Autodesk Inventor part; units mm, degrees
ref_plane "YZ Plane" through (0, 0, 0) normal (1, 0, 0) x (0, 1, 0)
ref_plane "XZ Plane" through (0, 0, 0) normal (0, 1, 0) x (-1, 0, 0)
ref_plane "XY Plane" through (0, 0, 0) normal (0, 0, 1) x (1, 0, 0)
sketch "Sketch1" plane through (0, 0, 0) normal (0, 0, 1) x (1, 0, 0)
  line L0 (-23.5606, 6.7424) -> (-13.5606, 6.7424)
  line L1 (-13.5606, 6.7424) -> (-13.5606, -1.2576)
  line L2 (-13.5606, -1.2576) -> (-23.5606, -1.2576)
  line L3 (-23.5606, -1.2576) -> (-23.5606, 6.7424)
  point P0 (0, 0)
  dimension "d0" = 10
  dimension "d1" = 8
extrude "Extrusion1" add sketch "Sketch1" along normal blind 23
sketch "Sketch2" plane through (0, 0, 23) normal (0, 0, 1) x (1, 0, 0)
  line L0 (-23.5606, 6.7424) -> (-23.5606, -1.2576)
  point P0 (0, 0)
  point P1 (-18.5606, 2.7424)
  dimension "d4" = 5
hole "Hole1" at (-18.5606, 2.7424, 23) direction (0, 0, -1) diameter 3 depth 8 tip angle 118
sketch "Sketch3" plane through (-13.5606, -1.2576, 0) normal (1, 0, 0) x (0, 0, -1)
  line L0 (0, 8) -> (-3, 8)
  line L1 (-3, 8) -> (-3, 13)
  line L2 (-3, 13) -> (0, 13)
  line L3 (0, 13) -> (0, 8)
  line L4 (0, 0) -> (-23, 0)
  point P0 (0, 1.2576)
  dimension "d12" = 13
  dimension "d13" = 3
extrude "Extrusion2" add sketch "Sketch3" against normal blind 10
chamfer "Chamfer1" distance 3 angle 45 1 edges at (-18.5606, 6.7424, 3)
properties part number "ArOZ Portable Mount"
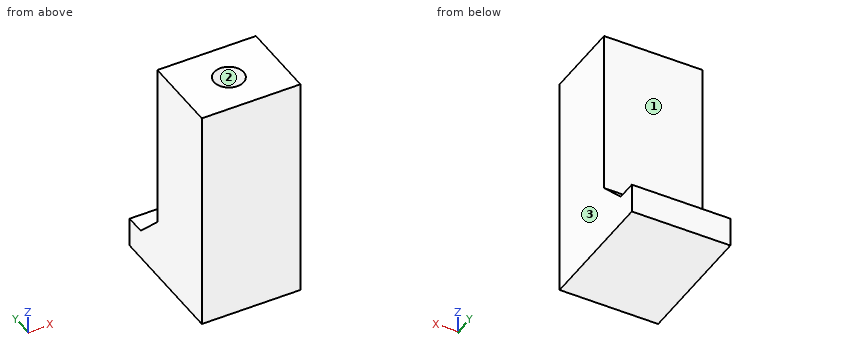
Could you check a few things on this model? Use its own coordinates, in mm. Face numbers are marked on the shaded views. Give positions to 0.01 mm unless a question says otherwise; leave off trailing zeros. Write each loop counter-clockwise with the first axis right and the second up, starting at its lowest first coordinate (ties: lowest second). Pieces come first, ordered by that corner, then holes. Notation, with made-up numbers: (-38, 45) - (-22, 45) arc R27 cw to (-22, 72) - close; hole circle Ø2 at (-40, -28.5). An arc over 180 degrees is marked (long way). Use CSV: the item, a comma, the result in double quotes. Start each with the question number.
Item 1: I'm going to push flat-ended pins straight in: pin 1 (1.5 mm diameter, centred on x = -21, y = 8.5, fed in from +Z); pin 2 (5 mm diameter, centred on x = -18, z = 11, fed in from +Y); pin 3 (2 mm diameter, centred on x = -16.5, y = 10.5, fed in from +Z). Where does each tip first touch, or does it pass through?
Item 2: I want a section at C-C, the plane y = 8.5. Please give me the cut outline in (x, z).
Item 3: I want a section at A-A, the plane x = -21. Please give me the cut outline in (y, z), then the cut area to 4 significant figures.
Item 4: If I drill on line 1 along X through (y, z) = (2.75, 17.5); line 2 along Y through (x, z) = (-16, 22.25); line 3 along Z through (x, y) = (-20, 11), over which ranges is the centre line in solid material (lowest first)?
Item 5: I want a section at B-B, the plane z = 19. Please give me the cut outline in (x, y), then the cut area to 3 significant figures.
Item 6: I want a section at D-D, the plane z = 9.25. Please give me the cut outline in (x, y).
Item 7: If we mould it in two halves opening along X, with no side actions, what happens to the marked faces 1, 2 and 3? For each: pulls with the +X half, pulls with the -X half, needs draft (parallel to the pull), parting line crosses it, or undercut.
Findings:
1,pin 1,"stops at z = 4.99"
1,pin 2,"stops at y = 6.74"
1,pin 3,"stops at z = 3.24"
2,outline,"(-23.56, 0) - (-13.56, 0) - (-13.56, 4.24) - (-23.56, 4.24) - close"
3,outline,"(-1.26, 0) - (11.74, 0) - (11.74, 3) - (9.74, 3) - (6.74, 6) - (6.74, 23) - (-1.26, 23) - close"
3,area,"203.5 mm2"
4,line 1,"x = -23.56 to -20.06, -17.06 to -13.56"
4,line 2,"y = -1.26 to 6.74"
4,line 3,"z = 0 to 3"
5,outline,"(-23.56, -1.26) - (-13.56, -1.26) - (-13.56, 6.74) - (-23.56, 6.74) - close; hole circle Ø3 at (-18.56, 2.74)"
5,area,"72.9 mm2"
6,outline,"(-23.56, -1.26) - (-13.56, -1.26) - (-13.56, 6.74) - (-23.56, 6.74) - close"
7,face 1,"needs draft"
7,face 2,"undercut"
7,face 3,"pulls with the +X half"
